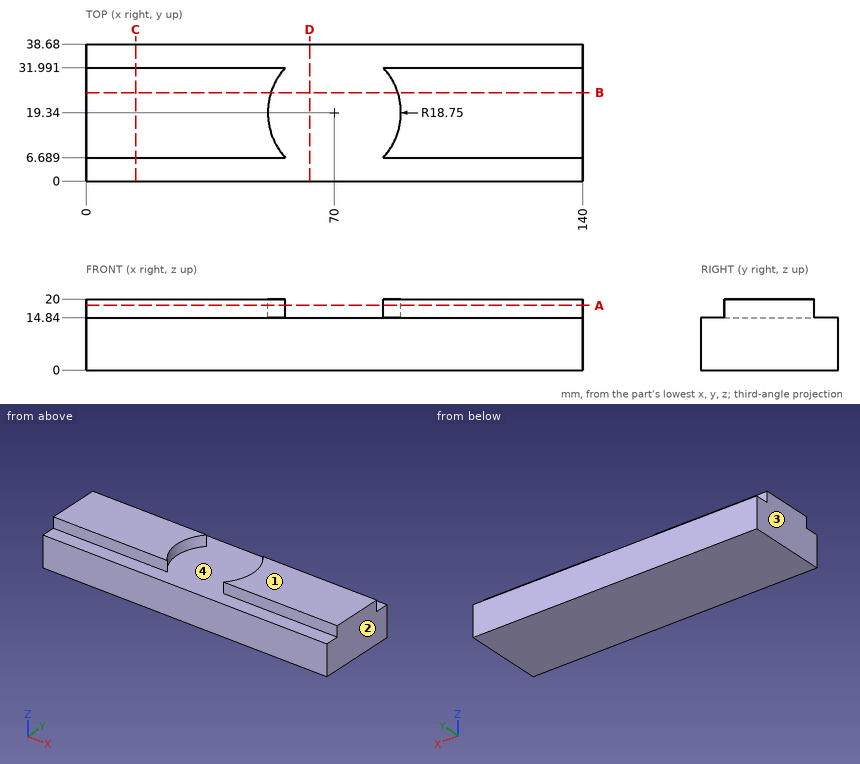
Drawing for the job (mm, zero at the part's lowest x, y, z). Round coordinates to 2 decimals unless told otherwise and drop trailing zeros. Write each loop counter-clockwise with the first axis right and the second up, starting at its lowest first coordinate (ties: lowest second). Pieces come first, ordered by that corner, then holes. Notation, with made-up numbers: (40.5, -5.5) - (50.5, -5.5) arc R27 ccw to (50.5, 33.5) - close; hole circle Ø11 at (61.5, -35). An arc over 180 degrees is marked (long way). Return JSON: item names as keys, results as strings. Group by question number.
Item 1: Probe probe 1 along Z at (x, y) = (15, 36); probe 2 along Y at (x, z) = (97, 17.75). List the from-to ranges inside material, lowest first.
Item 2: Flat gauge pins, fed straight in: pin 1 Ø2.5 at (x, z) = (111, 16.5) entering from -Y; pin 2 Ø2.5 at (x, z) = (14, 16.5) entering from +Y. Where does each tip first touch, or does it go through?
Item 3: Mould opens along X. For the marked faces 1, 2, 3 and 4 say: +X half, -X half, draft (parallel to the pull), parting line (faces both ways), or undercut.
Item 4: Band-saw the part on A-A on z = 18.25. List the corners of the cut face in (x, y).
Item 5: Band-saw the part on B-B on y = 25. List the corners of the cut face in (x, z) (1 decimal).
Item 6: Band-saw the part on C-C on x = 14. List the corners of the cut face in (y, z).
Item 7: Band-saw the part on D-D on x = 63. List the corners of the cut face in (y, z).
Resolved:
{
 "1": {"probe 1": "z = 0 to 14.84", "probe 2": "y = 6.69 to 31.99"},
 "2": {"pin 1": "stops at y = 6.69", "pin 2": "stops at y = 31.99"},
 "3": {"face 1": "draft", "face 2": "+X half", "face 3": "-X half", "face 4": "undercut"},
 "4": {"outline": "(0, 6.69) - (56.16, 6.69) arc R18.75 cw to (56.16, 31.99) - (0, 31.99) - close; (83.84, 6.69) - (140, 6.69) - (140, 31.99) - (83.84, 31.99) arc R18.75 cw to start"},
 "5": {"outline": "(0, 0) - (140, 0) - (140, 20) - (87.9, 20) - (87.9, 14.8) - (52.1, 14.8) - (52.1, 20) - (0, 20) - close"},
 "6": {"outline": "(0, 0) - (38.68, 0) - (38.68, 14.84) - (31.99, 14.84) - (31.99, 20) - (6.69, 20) - (6.69, 14.84) - (0, 14.84) - close"},
 "7": {"outline": "(0, 0) - (38.68, 0) - (38.68, 14.84) - (0, 14.84) - close"}
}
